Geometry check sheet. Reference: the model listing, model coordinates, mm. A direction names the side the tool comes from. Round coordinates to 2 decimals unless told otherwise and drop trailing zeros. Loops run counter-clockwise (first coordinate to the right, second up) from the corner with the lowest first, then second, coordinate; pieces in that order, holes last. Notation, with made-up numbers: M 1,-20.5 L 11,-20.5 A29 cw 11,0.5 Z; hole C 55,0 d10. An arc over 180 degrees is marked long. Write item = value, one per line.
from build123d import *

# Parameters (mm, degrees)
SKETCH_1_R      = 1.5
EXTRUDE_1_DEPTH = 2


with BuildPart() as part:
    # 草图1 → 凸台-拉伸1 (new body)
    with BuildSketch(Plane.XY):
        Polygon((-8.932938962, -10.700971973), (-10.932938962, -10.700971973), (-10.932938962, -5.700971973), (-8.932938962, -5.700971973), (-8.932938962, -2.200971973), (-6.432938962, -2.200971973), (-6.432938962, -3.700971973), (-3.832938962, -3.700971973), (-3.832938962, -2.200971973), (-0.832938962, -2.200971973), (-0.832938962, 0.799028027), (-3.832938962, 0.799028027), (-3.832938962, 2.299028027), (-6.432938962, 2.299028027), (-6.432938962, 0.799028027), (-8.932938962, 0.799028027), (-8.932938962, 4.299028027), (-10.932938962, 4.299028027), (-10.932938962, 9.299028027), (-8.932938962, 9.299028027), (-8.932938962, 11.299028027), (-7.932938962, 12.299028027), (16.567061038, 12.299028027), (16.567061038, 9.299028027), (18.567061038, 9.299028027), (18.567061038, 4.299028027), (16.567061038, 4.299028027), (16.567061038, 0.799028027), (14.067061038, 0.799028027), (14.067061038, 2.299028027), (11.467061038, 2.299028027), (11.467061038, 0.799028027), (8.467061038, 0.799028027), (8.467061038, -2.200971973), (11.467061038, -2.200971973), (11.467061038, -3.700971973), (14.067061038, -3.700971973), (14.067061038, -2.200971973), (16.567061038, -2.200971973), (16.567061038, -5.700971973), (18.567061038, -5.700971973), (18.567061038, -10.700971973), (16.567061038, -10.700971973), (16.567061038, -34.700971973), (4.222987954, -34.700971973), (3.817061038, -35.455763704), (3.411134121, -34.700971973), (-8.932938962, -34.700971973), align=None)
        with Locations((3.817061038, -5.700971973)):
            Circle(SKETCH_1_R, mode=Mode.SUBTRACT)
        with Locations((3.817061038, 3.799028027)):
            Circle(SKETCH_1_R, mode=Mode.SUBTRACT)
        with Locations((3.817061038, -31.692801434)):
            Circle(SKETCH_1_R, mode=Mode.SUBTRACT)
        with Locations((-3.832938962, 9.799028027)):
            Circle(SKETCH_1_R, mode=Mode.SUBTRACT)
        with Locations((11.467061038, 9.799028027)):
            Circle(SKETCH_1_R, mode=Mode.SUBTRACT)
        with BuildLine():
            Line((13.467061038, -32.842801434), (8.167061038, -32.842801434))
            ThreePointArc((8.167061038, -32.842801434), (7.690715441, -31.692801434), (8.167061038, -30.542801434))
            Line((8.167061038, -30.542801434), (13.467061038, -30.542801434))
            Line((13.467061038, -30.542801434), (13.467061038, -32.842801434))
        make_face(mode=Mode.SUBTRACT)
        with BuildLine():
            Line((-5.832938962, -30.542801434), (-0.532938962, -30.542801434))
            ThreePointArc((-0.532938962, -30.542801434), (-0.056593366, -31.692801434), (-0.532938962, -32.842801434))
            Line((-0.532938962, -32.842801434), (-5.832938962, -32.842801434))
            Line((-5.832938962, -32.842801434), (-5.832938962, -30.542801434))
        make_face(mode=Mode.SUBTRACT)
    extrude(amount=EXTRUDE_1_DEPTH)


solid = part.part
(1) Sectioned sample at D-D on y = -14. Record the cut outline in (x, z), then the cut area to 3 significant figures.
Result set:
outline = M -8.93,0 L 16.57,0 L 16.57,2 L -8.93,2 Z
area = 51.0 mm2
(2) Material ranges on line 1 along Y through (x, z) = (-5.5, 1.6); line 2 along Y through (x, z) = (9.25, 0.2); line 3 along X through (y, z) = (-3, 1.5), recorded low to high. Write a range as from..to.
Result set:
line_1 = -34.7..-32.84, -30.54..-3.7, 2.3..12.3
line_2 = -34.7..-32.84, -30.54..-2.2, 0.8..12.3
line_3 = -8.93..-6.43, -3.83..11.47, 14.07..16.57
(3) Depth check by flat-ended pin: pin 1 Ø1 at (x, z) = (-10, 1) entering from -Y; pin 2 Ø10 at (x, y) = (-1.5, -14) entering from -Z; pin 3 Ø1 at (y, z) = (-32, 1) entering from -X; pin 4 Ø2.5 at (x, y) = (3.82, 3.8) entering from +Z. Enter the tip coordinate at first touch or a pass-through.
Result set:
pin_1 = -10.7
pin_2 = 0
pin_3 = -8.93
pin_4 = through
(4) Release check for a two-part mould opening along Y. For faces 1 (the flat face through (18, -10.701, 1)), 2 (the flat face through (-0.833, -1, 1)), 3 (the flat face through (18, 9.299, 1)) record: released by +Y, released by -Y, zero draft, split by the parting line, or undercut.
Result set:
face_1 = released by -Y
face_2 = undercut
face_3 = released by +Y
(5) Sectioned sample at C-C on x = 6.75. Record the cut outline in (y, z).
Result set:
outline = M -34.7,0 L 12.3,0 L 12.3,2 L -34.7,2 Z
(6) Tool access check on faces 4 (the flat face through (16.567, -23, 1)), 5 (the flat face through (11.467, -3, 1)), 6 (the flat face through (16.567, 11, 1)), 7 (the flat face through (10, 0.799, 1)), 8 (the flat face through (-8.933, 3, 1)). Record the directions out of +Z, -Z, +X, -X, +Y, -Y that give a thin tool (end or side, any length) a straight path to the whole face; none if there is none.
Result set:
face_4 = +Z, -Z, +X, -Y
face_5 = +Z, -Z
face_6 = +Z, -Z, +X, +Y
face_7 = +Z, -Z, +X
face_8 = +Z, -Z, -X
(7) Sectioned sample at B-B on x = 10.5. Record the cut outline in (y, z), then the cut area to 3 significant figures.
Result set:
outline = M -34.7,0 L -32.84,0 L -32.84,2 L -34.7,2 Z; M -30.54,0 L -2.2,0 L -2.2,2 L -30.54,2 Z; M 0.8,0 L 8.65,0 L 8.65,2 L 0.8,2 Z; M 10.95,0 L 12.3,0 L 12.3,2 L 10.95,2 Z
area = 78.8 mm2
(8) Sectioned sample at A-A on y = -3. Record the cut outline in (x, z), then the cut area to 3 significant figures.
Result set:
outline = M -8.93,0 L -6.43,0 L -6.43,2 L -8.93,2 Z; M -3.83,0 L 11.47,0 L 11.47,2 L -3.83,2 Z; M 14.07,0 L 16.57,0 L 16.57,2 L 14.07,2 Z
area = 40.6 mm2
